from build123d import *

# Parameters (mm, degrees)
SKETCH_1_W          = 5
SKETCH_1_H          = 20
EXTRUDE_1_DEPTH     = 378
CUT_EXTRUDE_1_DEPTH = 6
SKETCH_3_R          = 2.5
CUT_EXTRUDE_2_DEPTH = 6
SKETCH_4_R          = 35
CUT_EXTRUDE_3_DEPTH = 6
CUT_EXTRUDE_4_DEPTH = 6
CUT_EXTRUDE_5_DEPTH = 6


with BuildPart() as part:
    # Эскиз1 → Бобышка-Вытянуть1 (new body)
    with BuildSketch(Plane(origin=(0, 0, 0), x_dir=(1, 0, 0), z_dir=(0, 1, 0))):
        with Locations((2.5, -10)):
            Rectangle(SKETCH_1_W, SKETCH_1_H)
    extrude(amount=EXTRUDE_1_DEPTH)

    # Эскиз2 → Вырез-Вытянуть1 (cut, through all)
    with BuildSketch(Plane.ZY):
        with BuildLine():
            Line((0, 10), (0, -2))
            Line((0, -2), (20, -2))
            Line((20, -2), (20, 10))
            ThreePointArc((20, 10), (10, 0), (0, 10))
        make_face()
    extrude(amount=-CUT_EXTRUDE_1_DEPTH, mode=Mode.SUBTRACT)

    # Эскиз3 → Вырез-Вытянуть2 (cut, through all)
    with BuildSketch(Plane.ZY):
        with Locations((10, 10)):
            Circle(SKETCH_3_R)
    extrude(amount=-CUT_EXTRUDE_2_DEPTH, mode=Mode.SUBTRACT)

    # Эскиз4 → Вырез-Вытянуть3 (cut, through all)
    with BuildSketch(Plane.ZY):
        with Locations((-27.5, 343)):
            Circle(SKETCH_4_R)
    extrude(amount=-CUT_EXTRUDE_3_DEPTH, mode=Mode.SUBTRACT)

    # Эскиз5 → Вырез-Вытянуть4 (cut, through all)
    with BuildSketch(Plane.ZY):
        with BuildLine():
            Line((0, 381.729833462), (20, 378))
            Line((20, 378), (20, 343))
            ThreePointArc((20, 343), (14.70485754, 364.794494718), (0, 381.729833462))
        make_face()
    extrude(amount=-CUT_EXTRUDE_4_DEPTH, mode=Mode.SUBTRACT)

    # Эскиз6 → Вырез-Вытянуть5 (cut, through all)
    with BuildSketch(Plane(origin=(5, 0, 0), x_dir=(0, 0, -1), z_dir=(1, 0, 0))):
        with BuildLine():
            Line((-16, 23.61), (-20, 23.61))
            Line((-20, 23.61), (-20, 19.51))
            Line((-20, 19.51), (-20, 14.520650354))
            ThreePointArc((-20, 14.520650354), (-17.967405564, 17.546968146), (-15.055614801, 19.740484516))
            ThreePointArc((-15.055614801, 19.740484516), (-14.008454527, 22.046052085), (-16, 23.61))
        make_face()
    extrude(amount=-CUT_EXTRUDE_5_DEPTH, mode=Mode.SUBTRACT)


solid = part.part
Part model, mm, in its own coordinate system. Coordinates: 2 decimals unless noted, no trailing zeros. Write each loop counter-clockwise with the first axis right and the second up, starting at its lowest first coordinate (ties: lowest second). Pieces come first, ordered by that corner, then holes. Notation, with made-up numbers: (28.5, -13.5) - (41.5, -13.5) arc R24 cw to (41.5, 25.5) - close; hole circle Ø9 at (33, 13). An arc over 180 degrees is marked (long way). Put each result on its own line as item: value.
1. Band-saw the part on A-A (x = 1.55). Write the cut outline in (y, z).
Final values:
outline: (10, 0) - (321.35, 0) arc R35 cw to (364.65, 0) - (378, 0) - (378, 4.61) arc R47.5 ccw to (343, 20) - (23.61, 20) - (23.61, 16) arc R2.05 cw to (19.74, 15.06) arc R10.97 ccw to (14.52, 20) - (10, 20) arc R10 ccw to start; hole circle Ø5 at (10, 10)
2. Flat gauge pin, fed straight in: pin 1 Ø2 at (x, z) = (3.5, 18) entering from -Y. Where does the tip first touch, or does it go through?
Final values:
pin 1: stops at y = 2.86
3. Probe line 1 along Y through (x, z) = (3.6, 10); line 2 along Y through (x, z) = (4.7, 14.75). List the from-to ranges inside material, lowest first. Write a range as [from, to].
Final values:
line 1: y = [0, 7.5], [12.5, 372.15]
line 2: y = [1.2, 19.94], [23.18, 364.71]
4. Two-plate mould, pull along Y, no slides. Class faces 1 (the cylindrical face through (2, 0, 10)), 2 (the flat face through (0, 186, 10)), 3 (the cylindrical face through (2.5, 342.7, 7.5)), 4 (the cylindrical face through (2.465, 361.864, 16.094)): +Y half, -Y half, draft (parallel to the pull), parting line (faces both ways), or undercut.
Final values:
face 1: -Y half
face 2: draft
face 3: undercut
face 4: +Y half
